Input: part model. Units: mm. Frame: model coordinates. Face numbers are marked on the shaded views. A direction names the side the tool comes from. Give positions to 0.01 mm unless a question says otherwise; leave off trailing zeros. Order: outer loops, then holes, each group sorted by start corner. A loop starts at its lowest first (then second) coordinate and runs counter-clockwise, first axis right, second up.
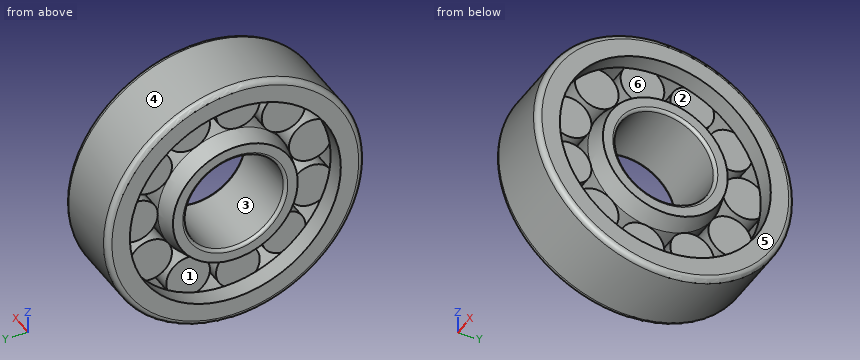
```python
from build123d import *

# Parameters (mm, degrees)
SKETCH2_W               = 7.5
SKETCH2_H               = 4.41
CIRCULAR_PATTERN1_COUNT = 11
FILLET1_R               = 1.1
FILLET2_R               = 0.6


with BuildPart() as part:
    # Sketch1 → Revolve1 (revolve)
    with BuildSketch(Plane.XY):
        Polygon((-7.5, 10), (7.5, 10), (7.5, 12.595190528), (3.75, 13.6), (-3.75, 13.6), (-7.5, 12.595190528), align=None)
    revolve(axis=Axis((-10.137871204, 0, 0), (1, 0, 0)))

    # Sketch2 → Revolve2 (revolve)
    with BuildSketch(Plane.XY):
        with Locations((0, 15.795)):
            Rectangle(SKETCH2_W, SKETCH2_H)
    revolve2 = revolve(axis=Axis((-7.422783257, 18, 0), (1, 0, 0)))

    # Sketch3 → Revolve3 (revolve)
    with BuildSketch(Plane.XY):
        Polygon((-7.5, 26), (7.5, 26), (7.5, 21.28), (3.74, 21.28), (3.74, 22.4), (-3.74, 22.4), (-3.74, 21.28), (-7.5, 21.28), align=None)
    revolve(axis=Axis((-9.082213196, 0, 0), (1, 0, 0)))

    # Circular-Pattern1: Revolve2 ×11 about axis
    circular_pattern1_axis = Axis((0, 0, 0), (1, 0, 0))
    for i in range(1, CIRCULAR_PATTERN1_COUNT):
        add(revolve2.rotate(circular_pattern1_axis, i * 360 / CIRCULAR_PATTERN1_COUNT))

    # Fillet1
    fillet1_edges = [part.edges().sort_by_distance(p)[0] for p in [
        (-7.5, -26, 0),
        (7.5, -26, 0),
    ]]
    fillet(fillet1_edges, radius=FILLET1_R)

    # Fillet2
    fillet2_edges = [part.edges().sort_by_distance(p)[0] for p in [
        (7.5, -10, 0),
        (-7.5, -10, 0),
    ]]
    fillet(fillet2_edges, radius=FILLET2_R)


solid = part.part
```
1) Cut plane A-A (x = 4.5). Return the cut outline in (y, z).
2) First-contact query: P1, Ø2.5, axis at y = -11.5, z = -13.5, coming from the +X side; P2, Ø2.5, axis at y = -13, z = 12.5, coming from the -X side; P3, Ø2, axis at x = -2, y = 1.5, coming from the +Z side. Flat tips, straight axial feed; report the tip coordinate or a pass-through.
3) Cut plane B-B (y = 18). Count the separate pieces of the cut face and the enclosed holes in it, then the cut area to 3 significant figures.
4) Line query: probe 1 along Z at (x, y) = (1, 0); probe 2 along Z at (x, y) = (5.85, 0); probe 3 along Y at (x, z) = (-0.5, 17). Output: solid intervals per line, ascending.
5) Reachability of the marked faces 1, 2 and 3 from +Z, -Z, +X, -X, +Y, -Y: full face, straight path, thin tool, end or side. Return the list, or none.
6) Pull-direction query (Z, two-part tool) for the marked faces 4, 5 and 6; classes: pulls with the +Z half, pulls with the -Z half, needs draft (parallel to the pull), parting line crosses it, or undercut.
Geometry says:
1. outline: circle Ø52 at (0, 0); circle Ø26.8 at (0, 0); hole circle Ø42.56 at (0, 0); hole circle Ø20 at (0, 0)
2. P1: stops at x = 3.75
2. P2: stops at x = -3.75
2. P3: stops at z = 26
3. separate pieces: 3
3. enclosed holes: 2
3. area: 358 mm2
4. probe 1: z = -26 to -22.4, -21.41 to -14.23, -13.6 to -10, 10 to 13.6, 14.23 to 21.41, 22.4 to 26
4. probe 2: z = -26 to -21.28, -13.04 to -10, 10 to 13.04, 21.28 to 26
4. probe 3: y = -19.67 to -8.97, -6.9 to 1.77, 3.11 to 11.84, 14.59 to 19.67
5. face 1: -X
5. face 2: +X
5. face 3: +X, -X
6. face 4: parting line crosses it
6. face 5: needs draft
6. face 6: undercut
